Geometry check sheet. Reference: drawing and pictorial views, mm from the part's lowest x, y, z. A direction names the side the tool comes from. Coordinates: 2 decimals unless noted, no trailing zeros. Loops run counter-clockwise (first coordinate to the right, second up) from the corner with the lowest first, then second, coordinate; pieces in that order, holes last. Notation, with made-up numbers: (-2, 16.25) -> (20, 16.25) arc R18 cw to (20, 34.25) -> close; hole circle Ø8 at (-26, 77.25). An arc over 180 degrees is marked (long way). Use CSV: the item, a comma, the result in double quotes.
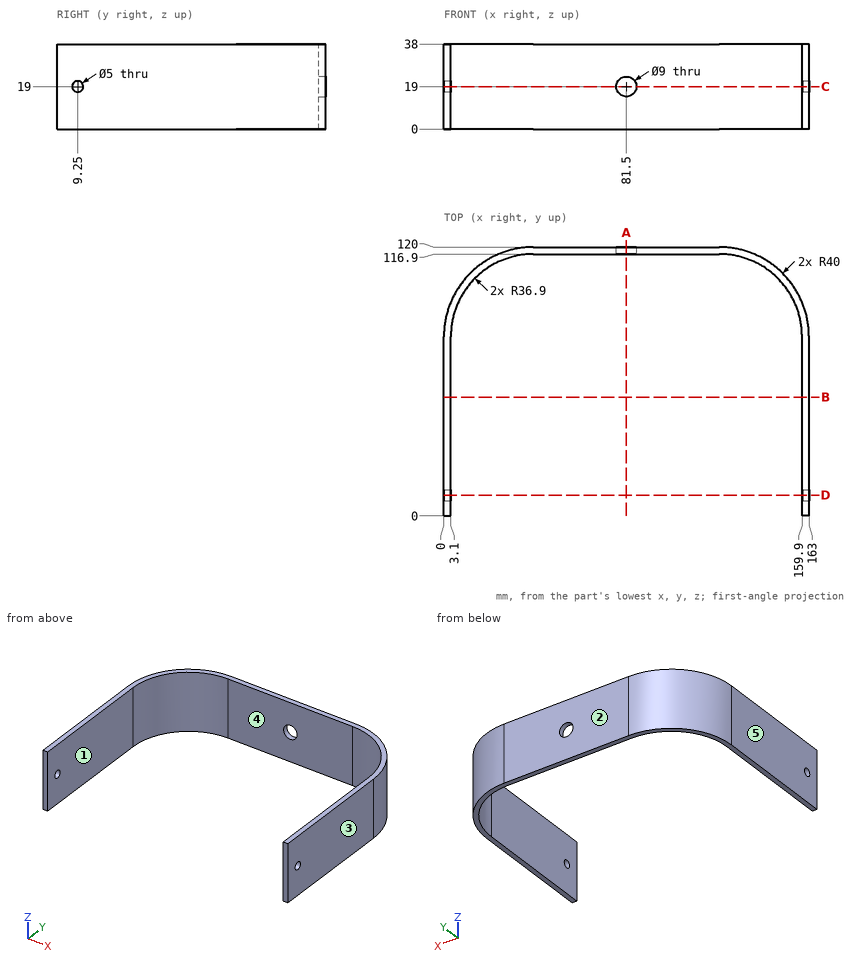
1) Cross-section at B-B on y = 53. Record the boundary of the cut face in (x, z), and give its area (3 significant figures).
Answer below:
outline,"(0, 0) -> (3.1, 0) -> (3.1, 38) -> (0, 38) -> close; (159.9, 0) -> (163, 0) -> (163, 38) -> (159.9, 38) -> close"
area,"236 mm²"
2) Cross-section at C-C on z = 19. Record the boundary of the cut face in (x, y), and give its area (3 significant figures).
Answer below:
outline,"(0, 0) -> (3.1, 0) -> (3.1, 6.75) -> (0, 6.75) -> close; (0, 11.75) -> (3.1, 11.75) -> (3.1, 80) arc R36.9 cw to (40, 116.9) -> (77, 116.9) -> (77, 120) -> (40, 120) arc R40 ccw to (0, 80) -> close; (86, 116.9) -> (123, 116.9) arc R36.9 cw to (159.9, 80) -> (159.9, 11.75) -> (163, 11.75) -> (163, 80) arc R40 ccw to (123, 120) -> (86, 120) -> close; (159.9, 0) -> (163, 0) -> (163, 6.75) -> (159.9, 6.75) -> close"
area,"1,070 mm²"
3) Cross-section at D-D on y = 9.25. Record the boundary of the cut face in (x, z), and give its area (3 significant figures).
Answer below:
outline,"(0, 0) -> (3.1, 0) -> (3.1, 16.5) -> (0, 16.5) -> close; (0, 21.5) -> (3.1, 21.5) -> (3.1, 38) -> (0, 38) -> close; (159.9, 0) -> (163, 0) -> (163, 16.5) -> (159.9, 16.5) -> close; (159.9, 21.5) -> (163, 21.5) -> (163, 38) -> (159.9, 38) -> close"
area,"205 mm²"
4) Draft check along X on the marked faces 3, 4 and 5. Enter one of: released by +X, released by -X, zero draft, split by the parting line, or undercut.
Answer below:
face 3,"released by +X"
face 4,"undercut"
face 5,"released by -X"
5) Access from +Z, -Z, +X, -X, +Y, -Y to the whole of each face (thin tool, end or side, straight path). Record for the marked faces 1 and 2.
Answer below:
face 1,"+Z, -Z, -Y"
face 2,"+Z, -Z, +X, -X, +Y"
6) Cross-section at A-A on x = 81.5. Record the boundary of the cut face in (y, z), and give its area (3 significant figures).
Answer below:
outline,"(116.9, 0) -> (120, 0) -> (120, 14.5) -> (116.9, 14.5) -> close; (116.9, 23.5) -> (120, 23.5) -> (120, 38) -> (116.9, 38) -> close"
area,"89.9 mm²"
7) Thickness scan on line 1 along X through (y, z) = (34.5, 23); line 2 along Z through (x, y) = (2, 9); line 3 along Y through (x, z) = (60.5, 7.5). Record the ranges inside material, lowest first. Write a range as from..to.
Answer below:
line 1,"x = 0..3.1, 159.9..163"
line 2,"z = 0..16.51, 21.49..38"
line 3,"y = 116.9..120"
8) Go/stop test with flat-tipped pins: pin 1 Ø3 at (y, z) = (103, 22.5) entering from -X; pin 2 Ø5 at (y, z) = (100, 29.5) entering from -X; pin 3 Ø19 at (x, z) = (92.5, 18) entering from -Y. Record where each tip stops, or that it passes through.
Answer below:
pin 1,"stops at x = 6.27"
pin 2,"stops at x = 4.03"
pin 3,"stops at y = 116.9"
